from build123d import *

# Parameters (mm, degrees)
SHAPE_DEPTH       = 6
SKETCH3_W         = 4.454383594
SKETCH3_H         = 6
LEVER_DEPTH       = 10
CUTS_START        = -9.408767
SKETCH2_R         = 1.5
CUTS_DEPTH        = 9.408767
LIMITS_1_DEPTH    = 4.454383594
LIMITS_START      = -4.454383594
LIMITS_2_DEPTH    = 4.454383594
ANGLE_FIX_1_DEPTH = 0.5


with BuildPart() as part:
    # Sketch1 → Shape (new body)
    with BuildSketch(Plane.XY):
        with BuildLine():
            Line((1.35, -7.59596768), (1.35, -8.6))
            Line((1.35, -8.6), (0.25, -8.6))
            Line((0.25, -8.6), (0.25, -14.6))
            Line((0.25, -14.6), (4.704383594, -14.6))
            Line((4.704383594, -14.6), (4.704383594, -8.5))
            ThreePointArc((4.704383594, -8.5), (0, 9.715), (-4.704383594, -8.5))
            Line((-4.704383594, -8.5), (-4.704383594, -14.6))
            Line((-4.704383594, -14.6), (-0.25, -14.6))
            Line((-0.25, -14.6), (-0.25, -8.6))
            Line((-0.25, -8.6), (-1.35, -8.6))
            Line((-1.35, -8.6), (-1.35, -7.59596768))
            ThreePointArc((-1.35, -7.59596768), (0, 7.715), (1.35, -7.59596768))
        make_face()
    extrude(amount=SHAPE_DEPTH)

    # Sketch3 → Lever (add)
    with BuildSketch(Plane(origin=(0, 0, 0), x_dir=(-1, 0, 0), z_dir=(0, 0, -1))):
        with Locations((-2.477191797, -11.6)):
            Rectangle(SKETCH3_W, SKETCH3_H)
        with Locations((2.477191797, -11.6)):
            Rectangle(SKETCH3_W, SKETCH3_H)
    extrude(amount=LEVER_DEPTH)

    # Sketch2 → Cuts (cut)
    with BuildSketch(Plane(origin=(4.704383594, 0, 0), x_dir=(0, 0, -1), z_dir=(1, 0, 0)).offset(CUTS_START)):
        with BuildLine():
            ThreePointArc((-3, -14.6), (-5.121320344, -13.721320344), (-6, -11.6))
            Line((-6, -11.6), (-6, -14.6))
            Line((-6, -14.6), (-3, -14.6))
        make_face()
        with BuildLine():
            Line((10, -8.6), (7, -8.6))
            ThreePointArc((7, -8.6), (9.121320344, -9.478679656), (10, -11.6))
            Line((10, -11.6), (10, -8.6))
        make_face()
        with BuildLine():
            ThreePointArc((10, -11.6), (9.121320344, -13.721320344), (7, -14.6))
            Line((7, -14.6), (10, -14.6))
            Line((10, -14.6), (10, -11.6))
        make_face()
        with Locations(Location((7, -11.6, 0), (0, 0, 90))):
            Circle(SKETCH2_R)
    extrude(amount=CUTS_DEPTH, mode=Mode.SUBTRACT)

    # Sketch5 → Limits 1 (add)
    with BuildSketch(Plane.ZY.offset(4.704383594)):
        with BuildLine():
            ThreePointArc((-4, -16.796152423), (-5.447085729, -17.395554958), (-7, -17.6))
            Line((-7, -17.6), (-4, -17.6))
            Line((-4, -17.6), (-4, -16.796152423))
        make_face()
        with BuildLine():
            Line((-7, -14.6), (-7, -17.6))
            ThreePointArc((-7, -17.6), (-5.447085729, -17.395554958), (-4, -16.796152423))
            Line((-4, -16.796152423), (-4, -14.6))
            Line((-4, -14.6), (-7, -14.6))
        make_face()
        with BuildLine():
            ThreePointArc((-12.437846722, -14.13570957), (-11.596266659, -15.456725658), (-10.441458618, -16.514912266))
            Line((-10.441458618, -16.514912266), (-8.720729309, -14.057456133))
            ThreePointArc((-8.720729309, -14.057456133), (-9.954423259, -12.120944533), (-9.457456133, -9.879270691))
            Line((-9.457456133, -9.879270691), (-12.437846722, -14.13570957))
        make_face()
        with BuildLine():
            Line((-12.898914751, -14.794182957), (-10.441458618, -16.514912266))
            ThreePointArc((-10.441458618, -16.514912266), (-11.596266659, -15.456725658), (-12.437846722, -14.13570957))
            Line((-12.437846722, -14.13570957), (-12.898914751, -14.794182957))
        make_face()
        with BuildLine():
            ThreePointArc((-10.441458618, -16.514912266), (-8.804234797, -17.322301704), (-7, -17.6))
            Line((-7, -17.6), (-7, -14.6))
            ThreePointArc((-7, -14.6), (-7.902117399, -14.461150852), (-8.720729309, -14.057456133))
            Line((-8.720729309, -14.057456133), (-10.441458618, -16.514912266))
        make_face()
        with BuildLine():
            Line((-4, -16.796152423), (-4, -17.6))
            Line((-4, -17.6), (-1, -14.6))
            Line((-1, -14.6), (-1.803847577, -14.6))
            ThreePointArc((-1.803847577, -14.6), (-2.757359313, -15.842640687), (-4, -16.796152423))
        make_face()
        with BuildLine():
            Line((-4, -14.6), (-4, -16.796152423))
            ThreePointArc((-4, -16.796152423), (-2.757359313, -15.842640687), (-1.803847577, -14.6))
            Line((-1.803847577, -14.6), (-4, -14.6))
        make_face()
    extrude(amount=-LIMITS_1_DEPTH)

    # Sketch6 → Limits 2 (add)
    with BuildSketch(Plane(origin=(4.704383594, 0, 0), x_dir=(0, 0, -1), z_dir=(1, 0, 0)).offset(LIMITS_START)):
        with BuildLine():
            Line((7, -14.6), (1, -14.6))
            Line((1, -14.6), (4, -17.6))
            Line((4, -17.6), (7, -17.6))
            ThreePointArc((7, -17.6), (8.804234797, -17.322301704), (10.441458618, -16.514912266))
            Line((10.441458618, -16.514912266), (12.898914751, -14.794182957))
            Line((12.898914751, -14.794182957), (9.457456133, -9.879270691))
            ThreePointArc((9.457456133, -9.879270691), (9.6610325, -12.98524584), (7, -14.6))
        make_face()
    extrude(amount=LIMITS_2_DEPTH)

    # Sketch7 → Angle fix 1 (cut)
    with BuildSketch(Plane.ZY.offset(4.704383594)):
        with BuildLine():
            Line((-8.312844754, -16.885973656), (-8.411191973, -17.443728451))
            Line((-8.411191973, -17.443728451), (-7.672586159, -17.573964585))
            Line((-7.672586159, -17.573964585), (-7.57423894, -17.01620979))
            ThreePointArc((-7.57423894, -17.01620979), (-7.474699486, -17.025839957), (-7.375, -17.033640938))
            Line((-7.375, -17.033640938), (-7.375, -17.6))
            Line((-7.375, -17.6), (-6.625, -17.6))
            Line((-6.625, -17.6), (-6.625, -15.886269614))
            ThreePointArc((-6.625, -15.886269614), (-8.113605815, -15.75603348), (-9.467894333, -15.124518373))
            Line((-9.467894333, -15.124518373), (-10.324759526, -16.608652423))
            Line((-10.324759526, -16.608652423), (-9.675240474, -16.983652423))
            Line((-9.675240474, -16.983652423), (-9.392060943, -16.493171087))
            ThreePointArc((-9.392060943, -16.493171087), (-9.301818164, -16.536264983), (-9.210799385, -16.57769474))
            Line((-9.210799385, -16.57769474), (-9.404505593, -17.109898171))
            Line((-9.404505593, -17.109898171), (-8.699736127, -17.366413278))
            Line((-8.699736127, -17.366413278), (-8.50602992, -16.834209847))
            ThreePointArc((-8.50602992, -16.834209847), (-8.409674955, -16.860978556), (-8.312844754, -16.885973656))
        make_face()
    angle_fix_1 = extrude(amount=-ANGLE_FIX_1_DEPTH, mode=Mode.SUBTRACT)

    # Angle fix 2: Angle fix 1 across plane
    add(angle_fix_1.mirror(Plane(origin=(0, 0, 0), x_dir=(0, 0, 1), z_dir=(1, 0, 0))), mode=Mode.SUBTRACT)


solid = part.part
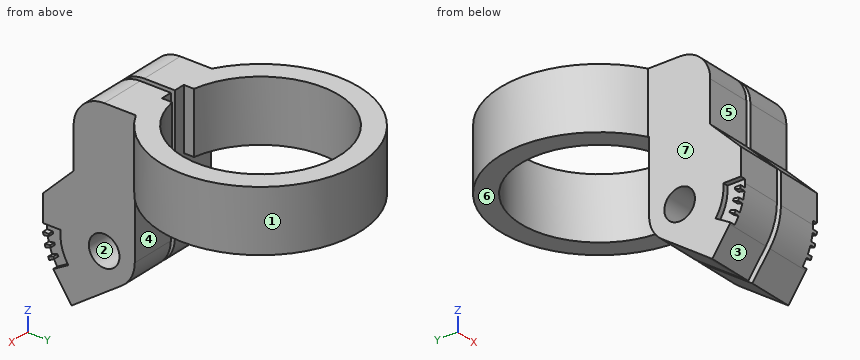
Source: CAD feature listing. Evaluate the final solid. Frame: model axes, mm. Face numbers are marked on the shaded views. A direction names the side the tool comes from. Give positions to 0.01 mm unless a question says otherwise; leave off trailing zeros. Order: outer loops, then holes, each group sorted by start corner. A loop starts at its lowest first (then second) coordinate and runs counter-clockwise, first axis right, second up. Notation, with made-up numbers: (53.25, 0.5) -> (92.25, 0.5) arc R25 cw to (92.25, 33.5) -> close; hole circle Ø1 at (39.5, -25). An arc over 180 degrees is marked (long way). Write item = value, one per line.
Q1. Cut plane C-C, the plane y = 4. Output: boundary loops of the cut face in (x, z).
Data:
outline = (-8.85, 0) -> (-6.6, 0) -> (-6.6, 6) -> (-8.85, 6) -> close; (6.6, 0) -> (8.85, 0) -> (8.85, 6) -> (6.6, 6) -> close
Q2. Pin query (flat end, axial travel): pin 1 (10 mm diameter, centred on x = 6.5, z = -5.5, fed in from +Y); pin 2 (10 mm diameter, centred on x = 2, z = 1.5, fed in from -Y); pin 3 (4.5 mm diameter, centred on y = -11.5, z = -0.5, fed in from -X). Return the tip coordinate at first contact, or that it passes through.
Data:
pin_1 = -8.6
pin_2 = -17.1
pin_3 = -4.7
Q3. Material intervals for line 1 (X direction, y = -11.25, z = 2.75); line 2 (X direction, y = 0, z = 2.4) (3 decimals); line 3 (Y direction, x = -1.6, z = -7), sorted ascending. Write a range as from..to.
Data:
line_1 = -4.7..-0.25, 0.25..4.7
line_2 = -9.715..-7.715, 7.715..9.715
line_3 = -17.6..-13.1, -10.1..-8.6
Q4. Set-up query: the marked faces 4, 5, 6 and 7. Return all of +Z, -Z, +X, -X, +Y, -Y with unobstructed straight access to the full face (end or side cutting, diameter ignored); none if empty.
Data:
face_4 = -Z
face_5 = +Z, +X, -X, -Y
face_6 = -Z, +X, -X, +Y
face_7 = +Z, -Z, -X, -Y
Q5. Pull-direction query (Y, two-part tool) for the marked faces 1, 2 and 3; classes: released by +Y, released by -Y, zero draft, split by the parting line, or undercut.
Data:
face_1 = split by the parting line
face_2 = undercut
face_3 = released by -Y
Q6. Cut plane B-B, the plane x = 3.5. Output: boundary loops of the cut face in (y, z).
Data:
outline = (-17.6, -7) arc R6 ccw to (-16.51, -10.44) -> (-14.79, -12.9) -> (-9.88, -9.46) arc R3 ccw to (-8.6, -7) -> (-8.6, 0) -> (-6.88, 0) -> (-6.88, 6) -> (-11.6, 6) arc R3 ccw to (-14.6, 3) -> (-14.6, -1) -> (-17.6, -4) -> close; (6.88, 0) -> (9.06, 0) -> (9.06, 6) -> (6.88, 6) -> close; hole circle Ø3 at (-11.6, -7)
Q7. Cut plane A-A, the plane y = 0. Output: boundary loops of the cut face in (x, z) (3 decimals).
Data:
outline = (-9.715, 0) -> (-7.715, 0) -> (-7.715, 6) -> (-9.715, 6) -> close; (7.715, 0) -> (9.715, 0) -> (9.715, 6) -> (7.715, 6) -> close
